```python
from build123d import *

# Parameters (mm, degrees)
BOSS_EXTRUDE1_DEPTH = 3.1115


with BuildPart() as part:
    # Sketch1 → Boss-Extrude1 (new body)
    with BuildSketch(Plane.XY):
        with BuildLine():
            Line((-11.346747426, -39.119290122), (11.669367426, -39.119721696))
            ThreePointArc((11.669367426, -39.119721696), (12.481628508, -35.808987017), (13.293765431, -39.119752155))
            Line((13.293765431, -39.119752155), (20.161810992, -39.119880937))
            Line((20.161810992, -39.119880937), (20.161869308, -36.009880938))
            Line((20.161869308, -36.009880938), (20.162213663, 35.990119062))
            Line((20.162213663, 35.990119062), (20.162213663, 39.100119058))
            Line((20.162213663, 39.100119058), (13.352237556, 39.100119058))
            Line((13.352237556, 39.100119058), (13.294498779, 39.100119058))
            ThreePointArc((13.294498779, 39.100119058), (12.482299776, 35.789369149), (11.670100774, 39.100119058))
            Line((11.670100774, 39.100119058), (-11.346014082, 39.100119058))
            ThreePointArc((-11.346014082, 39.100119058), (-12.158213085, 35.789369149), (-12.970412087, 39.100119058))
            Line((-12.970412087, 39.100119058), (-19.837839981, 39.100119058))
            Line((-19.837839981, 39.100119058), (-19.837939244, -36.009130904))
            Line((-19.837939244, -36.009130904), (-19.837956649, -39.119130904))
            Line((-19.837956649, -39.119130904), (-12.97114543, -39.119259663))
            ThreePointArc((-12.97114543, -39.119259663), (-12.158884348, -35.808524984), (-11.346747426, -39.119290122))
        make_face()
        Polygon((10.162043346, -0.008380505), (10.162043346, -1.913380505), (11.672043346, -1.913380505), (11.672043346, 1.896619495), (10.162043346, 1.896619495), align=None, mode=Mode.SUBTRACT)
        Polygon((-9.837956654, 1.896619495), (-9.837956654, -0.008380505), (-9.837956654, -1.913380505), (-11.347956654, -1.913380505), (-11.347956654, 1.896619495), align=None, mode=Mode.SUBTRACT)
    extrude(amount=BOSS_EXTRUDE1_DEPTH)


solid = part.part
```
Read the model definition and answer for the solid it produces. Units are mm, in the model's axes. A direction names the side the tool comes from. Give positions to 0.01 mm unless a question says otherwise; leave off trailing zeros. Order: outer loops, then holes, each group sorted by start corner. A loop starts at its lowest first (then second) coordinate and runs counter-clockwise, first axis right, second up. Notation, with made-up numbers: (33, -14) -> (90, -14) arc R22 cw to (90, 2) -> close; hole circle Ø9 at (50, -28.5). An arc over 180 degrees is marked (long way). Write item = value, one per line.
1. A cutting plane is placed at A-A, the plane z = 0.5. Write down the section's boundary in (x, y) (1 decimal), and give its area (3 significant figures).
Numbers:
outline = (-19.8, -39.1) -> (-13, -39.1) arc R1.8 cw (long way) to (-11.3, -39.1) -> (11.7, -39.1) arc R1.8 cw (long way) to (13.3, -39.1) -> (20.2, -39.1) -> (20.2, -36) -> (20.2, 36) -> (20.2, 39.1) -> (13.3, 39.1) arc R1.8 cw (long way) to (11.7, 39.1) -> (-11.3, 39.1) arc R1.8 cw (long way) to (-13, 39.1) -> (-19.8, 39.1) -> (-19.8, -36) -> close; hole (-11.3, -1.9) -> (-9.8, -1.9) -> (-9.8, 1.9) -> (-11.3, 1.9) -> close; hole (10.2, -1.9) -> (11.7, -1.9) -> (11.7, 1.9) -> (10.2, 1.9) -> close
area = 3,080 mm²
2. The mould has two halves that part along Y. Classify faces 1 (the face through (17, 39.1, 2)), 2 (the face through (-12.09, 35.79, 1.53)), 3 (the face through (0, 1, 3.112)): +Y half, -Y half, draft (parallel to the pull), parting line (faces both ways), or undercut.
Numbers:
face_1 = +Y half
face_2 = undercut
face_3 = draft
3. For faces 4 (the face through (11, 1.897, 2)), 5 (the face through (0, 39.1, 2)), determine the directions among +Z, -Z, +X, -X, +Y, -Y from which every point of the face is accessible in a straight line to the end or side of a thin tool.
Numbers:
face_4 = +Z, -Z
face_5 = +Z, -Z, +X, -X, +Y
4. A straight line is drawn through the part: line 1 along Y through (x, z) = (-11, 2.7). Find the intervals that lie inside material, in ascending order.
Numbers:
line_1 = -39.12 to -38.88, -36.25 to -1.91, 1.9 to 36.23, 38.86 to 39.1
5. Given pin 1 (5.5 mm diameter, centred on x = 12.48, y = 37.54, fed in from -Z), flat-ended and moving along its own axis, determine where the tip first touches the part or whether it passes through.
Numbers:
pin_1 = 0
